from build123d import *

# Parameters (mm, degrees)
F0_W     = 30
F0_H     = 10
F0_W_2   = 10
F2_R     = 2
F3_SIZE  = 2
F4_SIZE2 = 6
F4_SIZE  = 3


with BuildPart() as f1:
    # F0 (on Right) → F1 (revolve)
    with BuildSketch(Plane.YZ):
        Polygon((37.8557965517, 22.7), (27.8557965517, 22.7), (27.8557965517, 12.7), (31.5659119412, 12.7), (37.8557965517, 12.7), align=None)
        with Locations((52.8557965517, 17.7)):
            Rectangle(F0_W, F0_H)
        with Locations((32.8557965517, 27.7)):
            Rectangle(F0_W_2, F0_H)
    revolve(axis=Axis((0, 33.9278982759, 1.35), (0, 0.9992093063, 0.0397588012)))

    # F2
    f2_edges = [f1.edges().sort_by_distance(p)[0] for p in [
        (0, 39.539737, -19.620411),
    ]]
    fillet(f2_edges, radius=F2_R)

    # F3
    f3_edges = [f1.edges().sort_by_distance(p)[0] for p in [
        (0, 69.444891, -17.23677),
    ]]
    chamfer(f3_edges, length=F3_SIZE)

    # F4
    f4_edges = [f1.edges().sort_by_distance(p)[0] for p in [
        (0, 40.334284, -29.588796),
        (0, 30.365899, -30.383343),
    ]]
    f4_side = f1.faces().sort_by_distance((0, 35.350092, -29.98607))[0]
    chamfer(f4_edges, length=F4_SIZE, length2=F4_SIZE2, reference=f4_side)


solid = f1.part
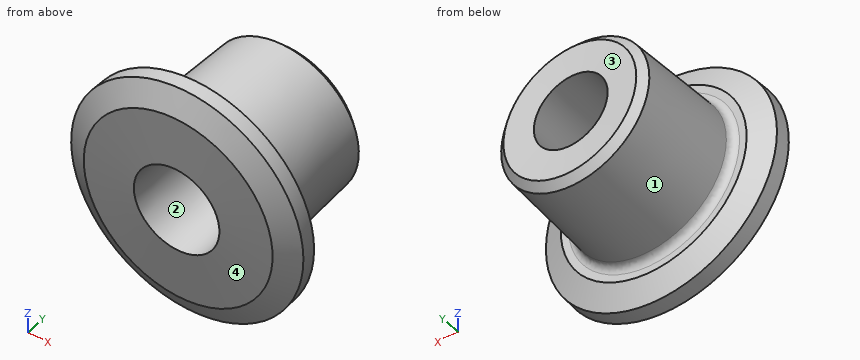
Verification items for the finished model (mm, model axes). Face numbers are marked on the shaded views. Coordinates: 2 decimals unless noted, no trailing zeros.
Item 1: Material ranges on L1, parallel to Z at x = 3, y = 62.5; L2, parallel to Z at x = -6.5, y = 54.5; L3, parallel to Y at x = 3, z = 15, recorded low to high.
Filled in:
L1: z = -17.57 to -7.31, 12.25 to 22.48
L2: z = -17.37 to -6.15, 10.46 to 21.64
L3: y = 27.87 to 67.87
Item 2: Depth check by flat-ended pin: pin 1 (2 mm diameter, centred on x = -17, y = 42, fed in from -Z); pin 2 (8 mm diameter, centred on x = -18, y = 54.5, fed in from +Z); pin 3 (1.5 mm diameter, centred on y = 37, z = -15.5, fed in from +X); pin 4 (5 mm diameter, centred on y = 41, z = 26.5, fed in from +X) (1 decimal). Enter the tip coordinate at first touch or a pass-through.
Filled in:
pin 1: stops at z = -12.05
pin 2: stops at z = 17.19
pin 3: stops at x = 26.74
pin 4: passes through
Item 3: Release check for a two-part mould opening along Z. For the marked faces 1, 2, 3 and 4 record: +Z half, -Z half, draft (parallel to the pull), parting line (faces both ways), or undercut.
Filled in:
face 1: parting line
face 2: undercut
face 3: +Z half
face 4: -Z half
